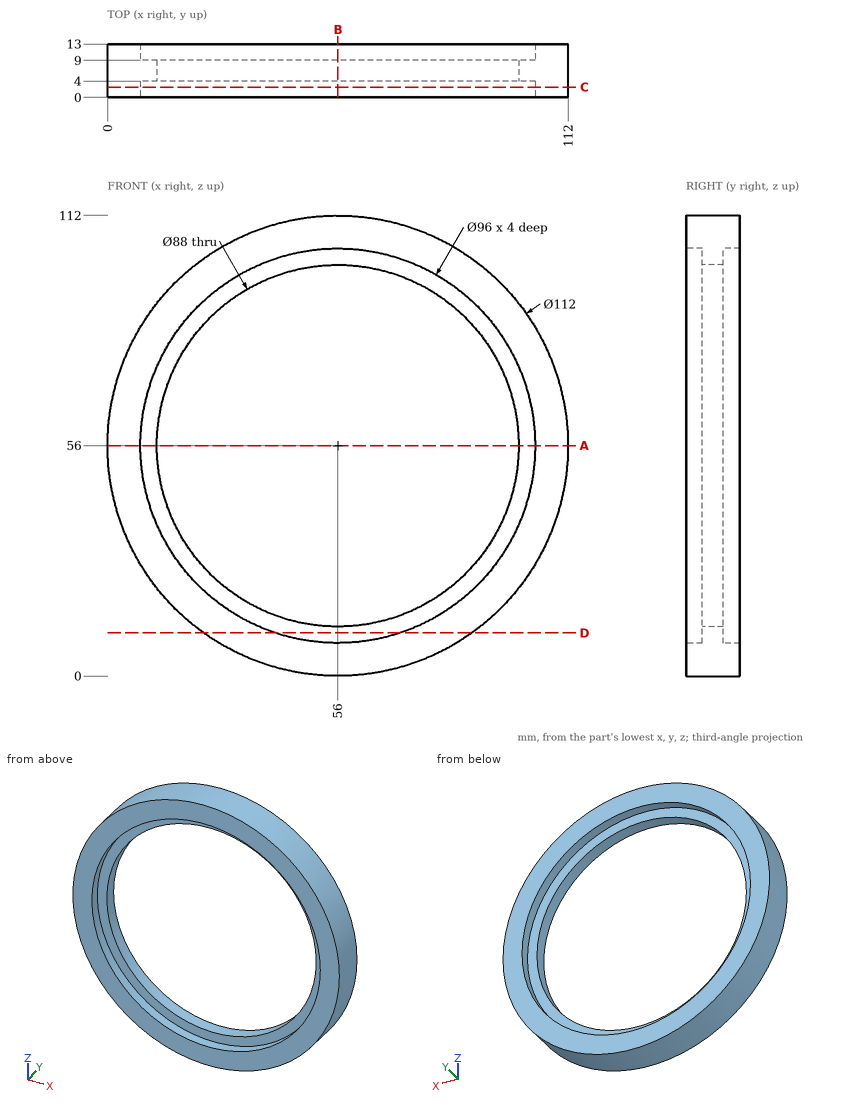
Design review of the part shown in the three views and the two pictorial views. Dimensions are in mm from the part's minimum x, y and z. Coordinates: 2 decimals unless noted, no trailing zeros. Loops run counter-clockwise (first coordinate to the right, second up) from the corner with the lowest first, then second, coordinate; pieces in that order, holes last.
(1) Consider section D-D, the plane z = 10.5. Give the boundary of the cut face in (x, y), plus the area to 3 significant figures.
Determined:
outline: (23.35, 0) - (40.71, 0) - (40.71, 4) - (71.29, 4) - (71.29, 0) - (88.65, 0) - (88.65, 13) - (71.29, 13) - (71.29, 9) - (40.71, 9) - (40.71, 13) - (23.35, 13) - close
area: 604 mm2
(2) Consider section C-C, the plane y = 2.5. Give the boundary of the cut face in (x, z), plus the area to 3 significant figures.
Determined:
outline: circle Ø112 at (56, 56); hole circle Ø96 at (56, 56)
area: 2,610 mm2
(3) Wall thickness on L1, parallel to X at y = 11.75, z = 57.5; L2, parallel to X at y = 6.2, z = 56; L3, parallel to Z at x = 56, y = 1.55: over which ranges is each line inside the solid? List them lowest first.
Determined:
L1: x = 0.02 to 8.02, 103.98 to 111.98
L2: x = 0 to 12, 100 to 112
L3: z = 0 to 8, 104 to 112
(4) Insertion check: P1, Ø5, axis at y = 7, z = 73, coming from the -X side; P2, Ø4, axis at x = 100, y = 4, coming from the -Z side; P3, Ø4, axis at y = 9, z = 52, coming from the +X side. Each pin has a flat end and moves straight along its axis. Give the tip position at first contact, or say it passes through.
Determined:
P1: stops at x = 1.91
P2: stops at z = 18.96
P3: stops at x = 111.96
(5) Consider section A-A, the plane z = 56. Give the boundary of the cut face in (x, y).
Determined:
outline: (0, 0) - (8, 0) - (8, 4) - (12, 4) - (12, 9) - (8, 9) - (8, 13) - (0, 13) - close; (100, 4) - (104, 4) - (104, 0) - (112, 0) - (112, 13) - (104, 13) - (104, 9) - (100, 9) - close
(6) Consider section B-B, the plane x = 56. Give the boundary of the cut face in (y, z), plus the area to 3 significant figures.
Determined:
outline: (0, 0) - (13, 0) - (13, 8) - (9, 8) - (9, 12) - (4, 12) - (4, 8) - (0, 8) - close; (0, 104) - (4, 104) - (4, 100) - (9, 100) - (9, 104) - (13, 104) - (13, 112) - (0, 112) - close
area: 248 mm2
